Model file for the job. Use its own axes, mm. A direction names the side the tool comes from. Give positions to 0.01 mm unless a question says otherwise; leave off trailing zeros. Loops run counter-clockwise (first coordinate to the right, second up) from the corner with the lowest first, then second, coordinate; pieces in that order, holes last. Notation, with made-up numbers: M -3,-35.75 L 30,-35.75 A17 cw 30,-16.75 Z; hole C -11.75,41 d3. An arc over 180 degrees is marked long. Use CSV: the item, a comma, the result in double quotes. Start each with the question number.
(1) Slice it at B-B on y = 0. List the corners of the cut face in (x, z).
(2) Flat gauge pins, fed straight in: P1, Ø4, axis at x = 0, y = 0, coming from the +Z side; P2, Ø6, axis at y = -4, z = 2, coming from the -X side; P3, Ø1.4, axis at y = 0, z = -3.5, coming from the -X side; P4, Ø1.5, axis at x = -6, z = -3.5, coming from the -Y side. Where does each tip first touch, or does it go through?
(3) Slice it at A-A on x = 0. List the corners of the cut face in (y, z).
(4) Slice it at C-C on z = -0.75. List the corners of the cut face in (x, y) (3 decimals), and give its area (3 significant figures).
(5) Tool access for faces 4 (the face through (-2, 0, -5)), 5 (the face through (0, -5, 2)), 6 (the face through (6.095, -0.256, -1.972)): list every direction of +Z, -Z, +X, -X, +Y, -Y with a clear straight run to the whole face (end or side of a thin tool).
(6) Slice it at D-D on z = 1. List the corners of the cut face in (x, y), and give its area (3 significant figures).
(7) Wall check: line 1 along Y through (x, z) = (0, 6); line 2 along Y through (x, z) = (0, -2); line 3 along Z through (x, y) = (-5, -4.25). Give the ranges that are in metal, low to high. Write a range as from..to.
(8) Two-plate mould, pull along Y, no slides. Class faces 1 (the face through (5.255, -0.221, -4.84)), 2 (the face through (-6.35, 0, -2)), 3 (the face through (-1.45, 0.06, 2.1)): pulls with the +Y half, pulls with the -Y half, needs draft (parallel to the pull), parting line crosses it, or undercut.
```python
from build123d import *

# Parameters (mm, degrees)
EXTRUDE_1_DEPTH     = 5
SKETCH_2_R          = 7.1
EXTRUDE_2_DEPTH     = 2
SKETCH_3_R          = 2.5
EXTRUDE_3_DEPTH     = 7
CHAMFER_1_SIZE      = 2
SKETCH_4_R          = 1.45
CUT_EXTRUDE_1_DEPTH = 30
CHAMFER_2_SIZE      = 1


with BuildPart() as part:
    # ｽｹｯﾁ1 → ﾎﾞｽ - 押し出し1 (new body)
    with BuildSketch(Plane.XY):
        with BuildLine():
            Line((-6.35, -0.875), (-6.036917674, -0.875))
            ThreePointArc((-6.036917674, -0.875), (6.1, 0), (-6.036917674, 0.875))
            Line((-6.036917674, 0.875), (-6.35, 0.875))
            Line((-6.35, 0.875), (-6.35, -0.875))
        make_face()
    extrude(amount=-EXTRUDE_1_DEPTH)

    # ｽｹｯﾁ2 → ﾎﾞｽ - 押し出し2 (add)
    with BuildSketch(Plane.XY):
        Circle(SKETCH_2_R)
    extrude(amount=EXTRUDE_2_DEPTH)

    # ｽｹｯﾁ3 → ﾎﾞｽ - 押し出し3 (add)
    with BuildSketch(Plane.XY.offset(2)):
        Circle(SKETCH_3_R)
    extrude(amount=EXTRUDE_3_DEPTH)

    # 面取り1
    chamfer_1_edges = [part.edges().sort_by_distance(p)[0] for p in [
        (-2.5, 0, 2),
    ]]
    chamfer(chamfer_1_edges, length=CHAMFER_1_SIZE)

    # ｽｹｯﾁ4 → ｶｯﾄ - 押し出し1 (cut)
    with BuildSketch(Plane.XY.offset(9)):
        Circle(SKETCH_4_R)
    extrude(amount=-CUT_EXTRUDE_1_DEPTH, mode=Mode.SUBTRACT)

    # 面取り2
    chamfer_2_edges = [part.edges().sort_by_distance(p)[0] for p in [
        (6.1, 0, -5),
    ]]
    chamfer(chamfer_2_edges, length=CHAMFER_2_SIZE)


solid = part.part
```
Reply:
1,outline,"M -7.1,0 L -6.35,0 L -6.35,-5 L -1.45,-5 L -1.45,9 L -2.5,9 L -2.5,4 L -4.5,2 L -7.1,2 Z; M 1.45,-5 L 5.1,-5 L 6.1,-4 L 6.1,0 L 7.1,0 L 7.1,2 L 4.5,2 L 2.5,4 L 2.5,9 L 1.45,9 Z"
2,P1,"stops at z = 9"
2,P2,"stops at x = -7.03"
2,P3,"stops at x = -6.35"
2,P4,"stops at y = -3.11"
3,outline,"M -7.1,0 L -6.1,0 L -6.1,-4 L -5.1,-5 L -1.45,-5 L -1.45,9 L -2.5,9 L -2.5,4 L -4.5,2 L -7.1,2 Z; M 1.45,-5 L 5.1,-5 L 6.1,-4 L 6.1,0 L 7.1,0 L 7.1,2 L 4.5,2 L 2.5,4 L 2.5,9 L 1.45,9 Z"
4,outline,"M -6.35,-0.875 L -6.037,-0.875 A6.1 ccw long -6.037,0.875 L -6.35,0.875 Z; hole C 0,0 d2.9"
4,area,"111 mm^2"
5,face 4,"-Z, +X, -X, +Y, -Y"
5,face 5,"+Z"
5,face 6,"-Z"
6,outline,"C 0,0 d14.2; hole C 0,0 d2.9"
6,area,"152 mm^2"
7,line 1,"y = -2.5..-1.45, 1.45..2.5"
7,line 2,"y = -6.1..-1.45, 1.45..6.1"
7,line 3,"z = 0..2"
8,face 1,"parting line crosses it"
8,face 2,"needs draft"
8,face 3,"undercut"
